The model under review builds one solid part; all positions refer to its coordinate system, in mm. A direction names the side the tool comes from. Coordinates: 2 decimals unless noted, no trailing zeros. Order: outer loops, then holes, each group sorted by start corner. A loop starts at its lowest first (then second) coordinate and runs counter-clockwise, first axis right, second up. Notation, with made-up numbers: M 78,-11 L 83,-11 A13 ccw 83,4 Z; hole C -1.5,-16.5 d6. An arc over 180 degrees is marked long. Answer in a Markdown table with one row per item.
from build123d import *

# Parameters (mm, degrees)
F0_R     = 1.5
F1_DEPTH = 4
F2_R     = 5


with BuildPart() as f1:
    # F0 (on Top) → F1 (new body)
    with BuildSketch(Plane.XY):
        with BuildLine():
            Line((-17.981, -11), (-10.3136468418, -11))
            Line((-10.3136468418, -11), (-16.1473234209, 0))
            Line((-16.1473234209, 0), (-20.1069034152, -7.4661972337))
            ThreePointArc((-20.1069034152, -7.4661972337), (-18.5534362632, -8.938009013), (-17.981, -11))
        make_face()
        with BuildLine():
            Line((-20.1069034152, -7.4661972337), (-16.1473234209, 0))
            Line((-16.1473234209, 0), (-20.1069034152, 7.4661972337))
            ThreePointArc((-20.1069034152, 7.4661972337), (-21.0153942484, 7.1182986291), (-21.981, 7))
            Line((-21.981, 7), (-21.981, -7))
            ThreePointArc((-21.981, -7), (-21.0153942484, -7.1182986291), (-20.1069034152, -7.4661972337))
        make_face()
        with BuildLine():
            Line((-16.1473234209, 0), (-10.3136468418, 11))
            Line((-10.3136468418, 11), (-17.981, 11))
            ThreePointArc((-17.981, 11), (-18.5534362632, 8.938009013), (-20.1069034152, 7.4661972337))
            Line((-20.1069034152, 7.4661972337), (-16.1473234209, 0))
        make_face()
        with BuildLine():
            ThreePointArc((-20.1069034152, 7.4661972337), (-18.5534362632, 8.938009013), (-17.981, 11))
            Line((-17.981, 11), (-20.481, 11))
            ThreePointArc((-20.481, 11), (-20.6956635987, 10.2267533799), (-21.2782137807, 9.6748239626))
            Line((-21.2782137807, 9.6748239626), (-20.1069034152, 7.4661972337))
        make_face()
        with BuildLine():
            Line((-20.481, 11), (-17.981, 11))
            ThreePointArc((-17.981, 11), (-24.8094271247, 13.8284271247), (-21.981, 7))
            Line((-21.981, 7), (-21.981, 9.5))
            ThreePointArc((-21.981, 9.5), (-23.0416601718, 12.0606601718), (-20.481, 11))
        make_face()
        with BuildLine():
            ThreePointArc((-21.981, 7), (-21.0153942484, 7.1182986291), (-20.1069034152, 7.4661972337))
            Line((-20.1069034152, 7.4661972337), (-21.2782137807, 9.6748239626))
            ThreePointArc((-21.2782137807, 9.6748239626), (-21.6188978432, 9.5443619859), (-21.981, 9.5))
            Line((-21.981, 9.5), (-21.981, 7))
        make_face()
        with BuildLine():
            Line((-21.2782137807, -9.6748239626), (-20.1069034152, -7.4661972337))
            ThreePointArc((-20.1069034152, -7.4661972337), (-21.0153942484, -7.1182986291), (-21.981, -7))
            Line((-21.981, -7), (-21.981, -9.5))
            ThreePointArc((-21.981, -9.5), (-21.6188978432, -9.5443619859), (-21.2782137807, -9.6748239626))
        make_face()
        with BuildLine():
            Line((-20.481, -11), (-17.981, -11))
            ThreePointArc((-17.981, -11), (-18.5534362632, -8.938009013), (-20.1069034152, -7.4661972337))
            Line((-20.1069034152, -7.4661972337), (-21.2782137807, -9.6748239626))
            ThreePointArc((-21.2782137807, -9.6748239626), (-20.6956635987, -10.2267533799), (-20.481, -11))
        make_face()
        with BuildLine():
            ThreePointArc((-21.981, -7), (-24.8094271247, -13.8284271247), (-17.981, -11))
            Line((-17.981, -11), (-20.481, -11))
            ThreePointArc((-20.481, -11), (-23.0416601718, -12.0606601718), (-21.981, -9.5))
            Line((-21.981, -9.5), (-21.981, -7))
        make_face()
        with BuildLine():
            Line((17.981, -11), (20.481, -11))
            ThreePointArc((20.481, -11), (20.6956635987, -10.2267533799), (21.2782137807, -9.6748239626))
            Line((21.2782137807, -9.6748239626), (20.1069034152, -7.4661972337))
            ThreePointArc((20.1069034152, -7.4661972337), (18.5534362632, -8.938009013), (17.981, -11))
        make_face()
        with BuildLine():
            ThreePointArc((21.2782137807, -9.6748239626), (21.6188978432, -9.5443619859), (21.981, -9.5))
            Line((21.981, -9.5), (21.981, -7))
            ThreePointArc((21.981, -7), (21.0153942484, -7.1182986291), (20.1069034152, -7.4661972337))
            Line((20.1069034152, -7.4661972337), (21.2782137807, -9.6748239626))
        make_face()
        with BuildLine():
            ThreePointArc((23.481, -11), (21.981, -12.5), (20.481, -11))
            Line((20.481, -11), (17.981, -11))
            ThreePointArc((17.981, -11), (21.981, -15), (25.981, -11))
            ThreePointArc((25.981, -11), (24.8094271247, -8.1715728753), (21.981, -7))
            Line((21.981, -7), (21.981, -9.5))
            ThreePointArc((21.981, -9.5), (23.0416601718, -9.9393398282), (23.481, -11))
        make_face()
        with BuildLine():
            ThreePointArc((17.981, 11), (18.5534362632, 8.938009013), (20.1069034152, 7.4661972337))
            Line((20.1069034152, 7.4661972337), (21.2782137807, 9.6748239626))
            ThreePointArc((21.2782137807, 9.6748239626), (20.6956635987, 10.2267533799), (20.481, 11))
            Line((20.481, 11), (17.981, 11))
        make_face()
        with BuildLine():
            ThreePointArc((20.1069034152, 7.4661972337), (21.0153942484, 7.1182986291), (21.981, 7))
            Line((21.981, 7), (21.981, 9.5))
            ThreePointArc((21.981, 9.5), (21.6188978432, 9.5443619859), (21.2782137807, 9.6748239626))
            Line((21.2782137807, 9.6748239626), (20.1069034152, 7.4661972337))
        make_face()
        with BuildLine():
            Line((21.981, 9.5), (21.981, 7))
            ThreePointArc((21.981, 7), (24.8094271247, 8.1715728753), (25.981, 11))
            ThreePointArc((25.981, 11), (21.981, 15), (17.981, 11))
            Line((17.981, 11), (20.481, 11))
            ThreePointArc((20.481, 11), (21.981, 12.5), (23.481, 11))
            ThreePointArc((23.481, 11), (23.0416601718, 9.9393398282), (21.981, 9.5))
        make_face()
        with BuildLine():
            ThreePointArc((20.1069034152, -7.4661972337), (21.0153942484, -7.1182986291), (21.981, -7))
            Line((21.981, -7), (21.981, 7))
            ThreePointArc((21.981, 7), (21.0153942484, 7.1182986291), (20.1069034152, 7.4661972337))
            Line((20.1069034152, 7.4661972337), (16.1473234209, 0))
            Line((16.1473234209, 0), (20.1069034152, -7.4661972337))
        make_face()
        with BuildLine():
            Line((10.3136468418, 11), (16.1473234209, 0))
            Line((16.1473234209, 0), (20.1069034152, 7.4661972337))
            ThreePointArc((20.1069034152, 7.4661972337), (18.5534362632, 8.938009013), (17.981, 11))
            Line((17.981, 11), (10.3136468418, 11))
        make_face()
        with BuildLine():
            Line((10.3136468418, -11), (17.981, -11))
            ThreePointArc((17.981, -11), (18.5534362632, -8.938009013), (20.1069034152, -7.4661972337))
            Line((20.1069034152, -7.4661972337), (16.1473234209, 0))
            Line((16.1473234209, 0), (10.3136468418, -11))
        make_face()
        with BuildLine():
            Line((2.1071307506, -11), (10.3136468418, -11))
            Line((10.3136468418, -11), (16.1473234209, 0))
            Line((16.1473234209, 0), (10.3136468418, 11))
            Line((10.3136468418, 11), (2.1071307506, 11))
            ThreePointArc((2.1071307506, 11), (8.6324928151, 7.1358298604), (11.2, 0))
            ThreePointArc((11.2, 0), (8.6324928151, -7.1358298604), (2.1071307506, -11))
        make_face()
        with BuildLine():
            Line((-10.3136468418, -11), (-2.1071307506, -11))
            ThreePointArc((-2.1071307506, -11), (-11.2, 0), (-2.1071307506, 11))
            Line((-2.1071307506, 11), (-10.3136468418, 11))
            Line((-10.3136468418, 11), (-16.1473234209, 0))
            Line((-16.1473234209, 0), (-10.3136468418, -11))
        make_face()
        with BuildLine():
            Line((3.5338027663, -23.7840965848), (10.3136468418, -11))
            Line((10.3136468418, -11), (2.1071307506, -11))
            ThreePointArc((2.1071307506, -11), (0, -11.2), (-2.1071307506, -11))
            Line((-2.1071307506, -11), (-10.3136468418, -11))
            Line((-10.3136468418, -11), (-3.5338027663, -23.7840965848))
            ThreePointArc((-3.5338027663, -23.7840965848), (-0.9656057516, -18.0282986291), (4, -21.91))
            ThreePointArc((4, -21.91), (3.8817013709, -22.8756057516), (3.5338027663, -23.7840965848))
        make_face()
        with BuildLine():
            Line((2.1071307506, 11), (10.3136468418, 11))
            Line((10.3136468418, 11), (3.5338027663, 23.7840965848))
            ThreePointArc((3.5338027663, 23.7840965848), (3.8817013709, 22.8756057516), (4, 21.91))
            ThreePointArc((4, 21.91), (-0.9656057516, 18.0282986291), (-3.5338027663, 23.7840965848))
            Line((-3.5338027663, 23.7840965848), (-10.3136468418, 11))
            Line((-10.3136468418, 11), (-2.1071307506, 11))
            ThreePointArc((-2.1071307506, 11), (0, 11.2), (2.1071307506, 11))
        make_face()
        with BuildLine():
            ThreePointArc((4, 21.91), (3.8817013709, 22.8756057516), (3.5338027663, 23.7840965848))
            ThreePointArc((3.5338027663, 23.7840965848), (0, 25.91), (-3.5338027663, 23.7840965848))
            ThreePointArc((-3.5338027663, 23.7840965848), (-0.9656057516, 18.0282986291), (4, 21.91))
        make_face()
        with Locations((0, 21.91)):
            Circle(F0_R, mode=Mode.SUBTRACT)
        with BuildLine():
            ThreePointArc((-3.5338027663, -23.7840965848), (0, -25.91), (3.5338027663, -23.7840965848))
            ThreePointArc((3.5338027663, -23.7840965848), (3.8817013709, -22.8756057516), (4, -21.91))
            ThreePointArc((4, -21.91), (-0.9656057516, -18.0282986291), (-3.5338027663, -23.7840965848))
        make_face()
        with Locations((0, -21.91)):
            Circle(F0_R, mode=Mode.SUBTRACT)
    extrude(amount=F1_DEPTH)

    # F2
    f2_edges = [f1.edges().sort_by_distance(p)[0] for p in [
        (-17.981, -11, 2),
        (-10.313647, -11, 2),
        (-21.981, 7, 2),
        (-21.981, -7, 2),
        (-17.981, 11, 2),
        (-10.313647, 11, 2),
        (10.313647, 11, 2),
        (17.981, 11, 2),
        (21.981, 7, 2),
        (21.981, -7, 2),
        (17.981, -11, 2),
        (10.313647, -11, 2),
    ]]
    fillet(f2_edges, radius=F2_R)


solid = f1.part
(1) Take a section at A-A (x = 0). Write out the cut boundary in (y, z).
Report:
| item | result |
|---|---|
| outline | M -25.91,0 L -23.41,0 L -23.41,4 L -25.91,4 Z; M -20.41,0 L -11.2,0 L -11.2,4 L -20.41,4 Z; M 11.2,0 L 20.41,0 L 20.41,4 L 11.2,4 Z; M 23.41,0 L 25.91,0 L 25.91,4 L 23.41,4 Z |
(2) To check wall thickness, follow line 1 (Y direction, x = 0, z = 3.05); line 2 (Y direction, x = -19, z = 3.3); line 3 (X direction, y = -10, z = 0.45). State the ranges of each line that lie inside material, in increasing order. Write a range as [from, to].
Report:
| item | result |
|---|---|
| line 1 | [-25.91, -23.41], [-20.41, -11.2], [11.2, 20.41], [23.41, 25.91] |
| line 2 | [-13.67, 13.67] |
| line 3 | [-25.85, -23.1], [-20.86, -5.04], [5.04, 20.86], [23.1, 25.85] |
(3) Take a section at D-D (z = 2.6). State how many separate pieces and enclosed holes the cut face has, then the cut area to 3 significant figures.
Report:
| item | result |
|---|---|
| separate pieces | 1 |
| enclosed holes | 7 |
| area | 1,080 mm^2 |
(4) The part is to be moulded in two halves that separate along X. For faces 6 (the cylindrical face through (16.82, 11.57, 2.03)), 7 (the flat face through (-21.981, 0, 2)), 8 (the flat face through (6, 10, 0)), say which applies: +X half, -X half, draft (parallel to the pull), parting line (faces both ways), or undercut.
Report:
| item | result |
|---|---|
| face 6 | undercut |
| face 7 | -X half |
| face 8 | draft |
(5) Take a section at B-B (y = -21.91). Write out the cut boundary in (x, z), then the cut area to 3 significant figures.
Report:
| item | result |
|---|---|
| outline | M -4.53,0 L -1.5,0 L -1.5,4 L -4.53,4 Z; M 1.5,0 L 4.53,0 L 4.53,4 L 1.5,4 Z |
| area | 24.2 mm^2 |
(6) Take a section at C-C (x = 6). Write out the cut boundary in (y, z), then the cut area to 3 significant figures.
Report:
| item | result |
|---|---|
| outline | M -19.13,0 L -9.46,0 L -9.46,4 L -19.13,4 Z; M 9.46,0 L 19.13,0 L 19.13,4 L 9.46,4 Z |
| area | 77.4 mm^2 |
(7) Insertion check: P1, Ø1.3, axis at x = 13.5, z = 3, coming from the -Y side; P2, Ø1, axis at x = 4, z = 3.5, coming from the +Y side; P3, Ø0.6, axis at x = -14, z = 1, coming from the +Y side. Each pin has a flat end and moves straight along its axis. Give the tip position at first contact, or say it passes through.
Report:
| item | result |
|---|---|
| P1 | y = -11.02 |
| P2 | y = 23.85 |
| P3 | y = 11 |
(8) Machinability: for faces 1 (the cylindrical face through (-0.325, 20.446, 1.972)), 2 (the flat face through (21.981, 0, 2)), 3 (the flat face through (14, -11, 2)), 4 (the flat face through (-14, 11, 2)), 5 (the cylindrical face through (-22.588, 5.904, 2.028)), which of the approach directions +Z, -Z, +X, -X, +Y, -Y give a long, thin tool a straight path to every point of the face, cutting with its end or side? Answer none if there is none.
Report:
| item | result |
|---|---|
| face 1 | +Z, -Z |
| face 2 | +Z, -Z, +X |
| face 3 | +Z, -Z, -Y |
| face 4 | +Z, -Z, +Y |
| face 5 | +Z, -Z, -X |
